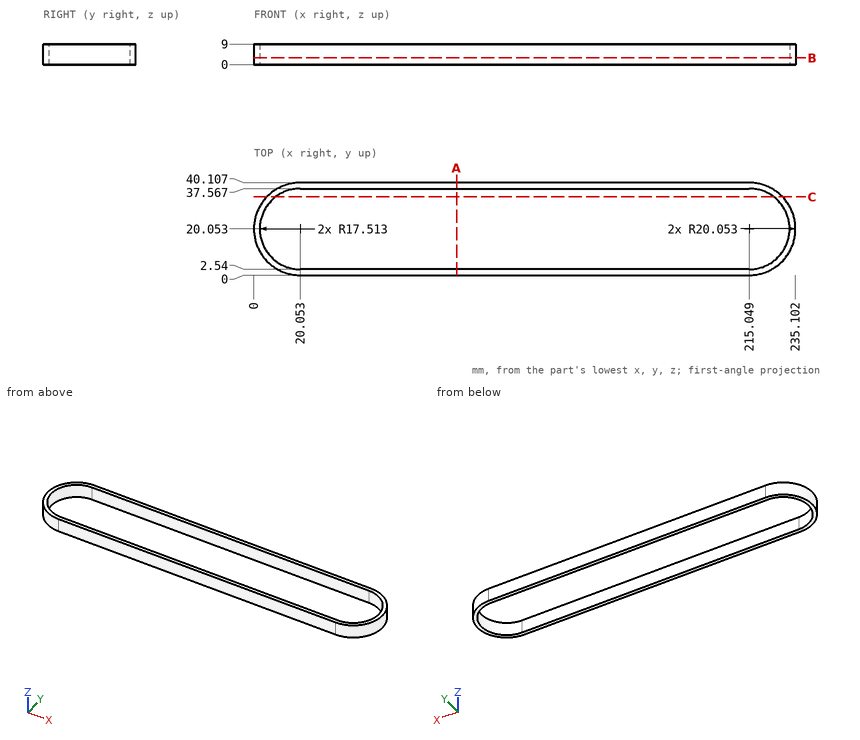
The figure shows three views and two pictorial views of one solid part (mm, origin at its lowest corner). Answer the questions. Round coordinates to 2 decimals unless told otherwise and drop trailing zeros. Order: outer loops, then holes, each group sorted by start corner. A loop starts at its lowest first (then second) coordinate and runs counter-clockwise, first axis right, second up.
Q1. A cutting plane is placed at A-A, the plane x = 88. Determine the outline of the cut face in (y, z).
Solution:
outline: (0, 0) - (2.54, 0) - (2.54, 9) - (0, 9) - close; (37.57, 0) - (40.11, 0) - (40.11, 9) - (37.57, 9) - close
Q2. Given pin 1 Ø5 at (y, z) = (10, 1.5) entering from -X; pin 2 Ø1 at (x, y) = (172.5, 5) entering from +Z; pin 3 Ø4 at (y, z) = (28, 3) entering from +X; pin 4 Ø1 at (y, z) = (5.5, 4) entering from +X (1 decimal), each flat-ended and moving along its own axis, determine where each tip first touches the part or whether it passes through.
Solution:
pin 1: stops at x = 1.48
pin 2: passes through
pin 3: stops at x = 234.2
pin 4: stops at x = 229.4
Q3. Find the intervals of material crossed by line 1 along Y through (x, z) = (132.5, 4.75); line 2 along X through (y, z) = (20, 7); line 3 along X through (y, z) = (19.5, 8.5) (1 decimal), in increasing order.
Solution:
line 1: y = 0 to 2.54, 37.57 to 40.11
line 2: x = 0 to 2.54, 232.56 to 235.1
line 3: x = 0 to 2.5, 232.6 to 235.1
Q4. A cutting plane is placed at C-C, the plane y = 34. Determine the outline of the cut face in (x, z).
Solution:
outline: (5.64, 0) - (9.46, 0) - (9.46, 9) - (5.64, 9) - close; (225.64, 0) - (229.46, 0) - (229.46, 9) - (225.64, 9) - close
Q5. A cutting plane is placed at B-B, the plane z = 3. Determine the outline of the cut face in (x, y), then the cut area to 3 significant figures.
Solution:
outline: (20.05, 0) - (215.05, 0) arc R20.05 ccw to (215.05, 40.11) - (20.05, 40.11) arc R20.05 ccw to start; hole (20.05, 2.54) - (215.05, 2.54) arc R17.51 ccw to (215.05, 37.57) - (20.05, 37.57) arc R17.51 ccw to start
area: 1,290 mm2
